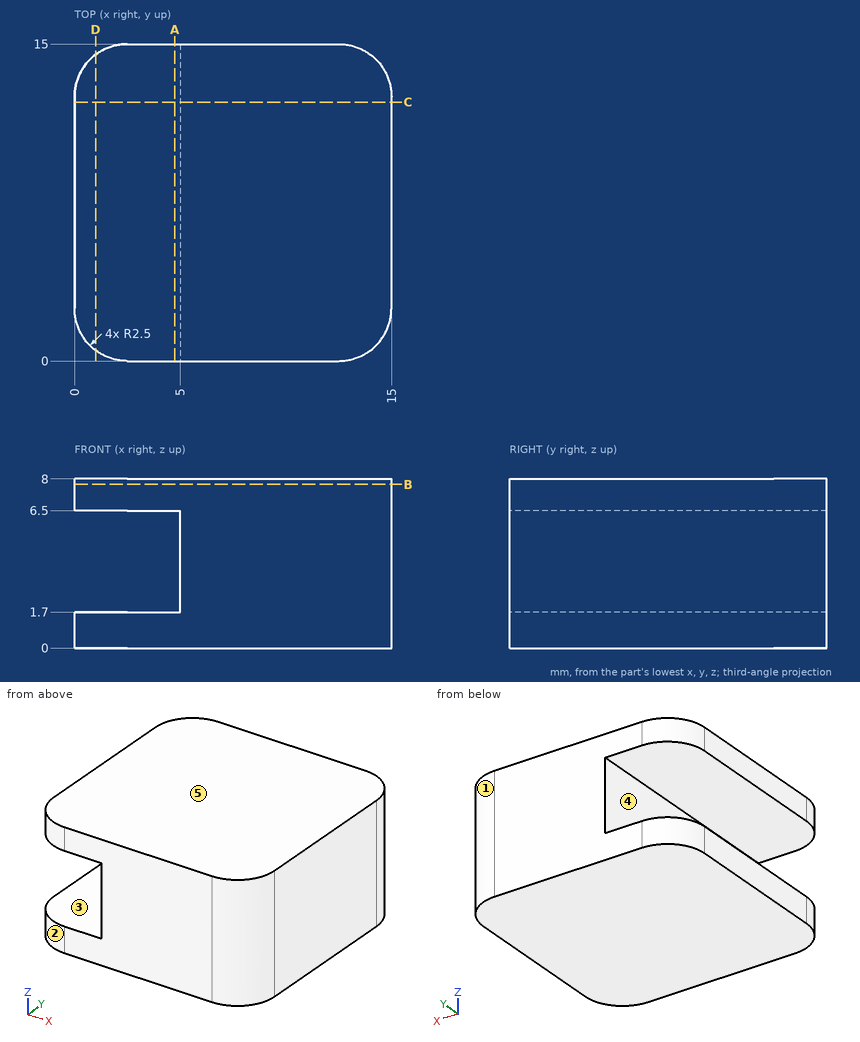
Job drawing, mm, ordinate dimensions from the low corner. One solid piece. A direction names the side the tool comes from. Round coordinates to 2 decimals unless told otherwise and drop trailing zeros. Write each loop counter-clockwise with the first axis right and the second up, starting at its lowest first coordinate (ties: lowest second). Pieces come first, ordered by that corner, then holes.
1) Mould opens along Y. For the marked faces 1, 2 and 3 say: +Y half, -Y half, draft (parallel to the pull), parting line (faces both ways), or undercut.
2) Band-saw the part on B-B, the plane z = 7.75. List the corners of the cut face in (x, y), and give its area (3 significant figures).
3) Drill centre lines: probe 1 along Z at (x, y) = (3, 9); probe 2 along X at (y, z) = (5.75, 1.75); probe 3 along Y at (x, z) = (14, 7.75). Where is each one in solid material? Low to high.
4) Band-saw the part on A-A, the plane x = 4.75. List the corners of the cut face in (y, z).
5) Band-saw the part on C-C, the plane y = 12.25. List the corners of the cut face in (x, z).
6) 3-axis set-ups, long thin cutter, end or side, ignore diameter. For the marked faces 4 and 5: which of +Z, -Z, +X, -X, +Y, -Y reach the whole face in a straight line?
7) Band-saw the part on D-D, the plane x = 1. List the corners of the cut face in (y, z), and give its area (3 significant figures).
Ans:
1. face 1: +Y half
1. face 2: -Y half
1. face 3: draft
2. outline: (0, 2.5) arc R2.5 ccw to (2.5, 0) - (12.5, 0) arc R2.5 ccw to (15, 2.5) - (15, 12.5) arc R2.5 ccw to (12.5, 15) - (2.5, 15) arc R2.5 ccw to (0, 12.5) - close
2. area: 220 mm2
3. probe 1: z = 0 to 1.7, 6.5 to 8
3. probe 2: x = 5 to 15
3. probe 3: y = 0.5 to 14.5
4. outline: (0, 0) - (15, 0) - (15, 1.7) - (0, 1.7) - close; (0, 6.5) - (15, 6.5) - (15, 8) - (0, 8) - close
5. outline: (0, 0) - (15, 0) - (15, 8) - (0, 8) - (0, 6.5) - (5, 6.5) - (5, 1.7) - (0, 1.7) - close
6. face 4: -X, +Y, -Y
6. face 5: +Z, +X, -X, +Y, -Y
7. outline: (0.5, 0) - (14.5, 0) - (14.5, 1.7) - (0.5, 1.7) - close; (0.5, 6.5) - (14.5, 6.5) - (14.5, 8) - (0.5, 8) - close
7. area: 44.8 mm2
